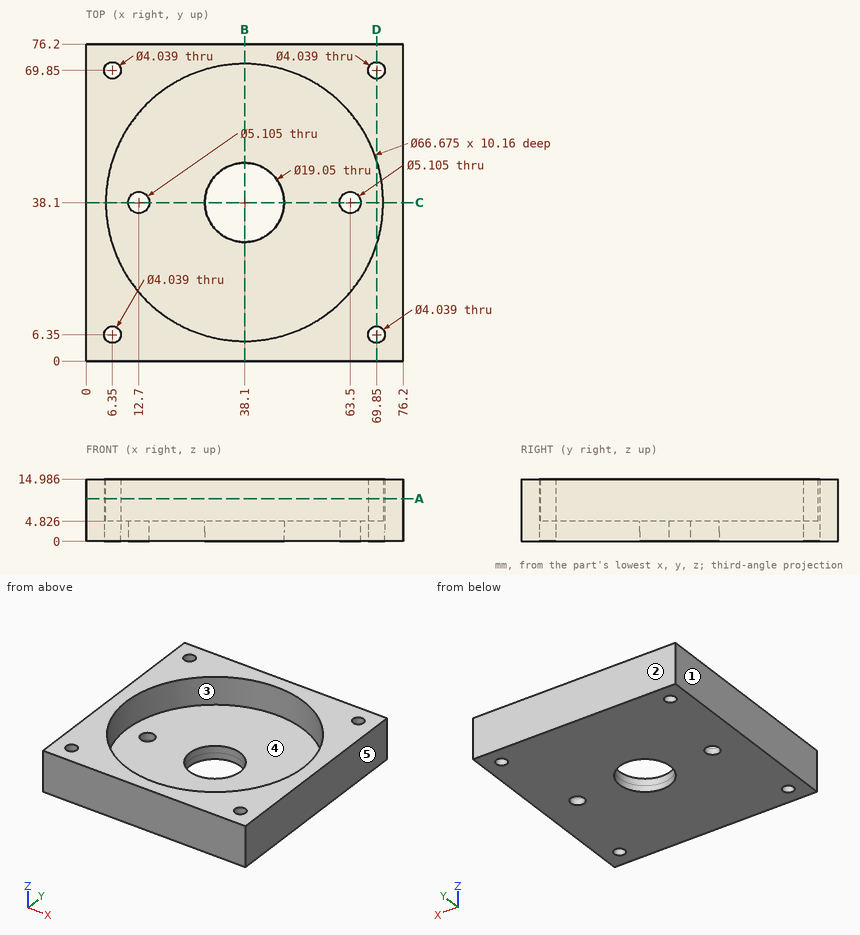
Part print with two shaded views. Sizes in mm from the minimum x, y, z corner. A direction names the side the tool comes from. Give positions to 0.01 mm unless a question says otherwise; leave off trailing zeros. Order: outer loops, then holes, each group sorted by start corner. A loop starts at its lowest first (then second) coordinate and runs counter-clockwise, first axis right, second up.
(1) Drill centre lines: L1, parallel to X at y = 69.85, z = 0.5; L2, parallel to Y at x = 63.5, z = 1.5; L3, parallel to Y at x = 38, z = 7.75. Where is each one in solid material? Low to high.
(2) Mould opens along X. For the marked faces 1, 2 and 3 say: released by +X, released by -X, zero draft, split by the parting line, or undercut.
(3) Flat gauge pins, fed straight in: pin 1 (8 mm diameter, centred on x = 18.5, z = 8, fed in from -Y); pin 2 (8 mm diameter, centred on x = 63.5, y = 38.1, fed in from +Z). Where does each tip first touch, or does it go through?
(4) Saw through at C-C, the plane y = 38.1. Give the cut face in (x, z) (1 decimal).
(5) Saw through at B-B, the plane x = 38.1. Give the cut face in (y, z) (1 decimal).
(6) Saw through at A-A, the plane z = 10.25. State how many separate pieces and enclosed holes the cut face has, then the cut area to 3 significant figures.
(7) Tool access for the marked faces 4 and 5: list every direction of +Z, -Z, +X, -X, +Y, -Y with a clear straight run to the whole face (end or side of a thin tool).
(8) Saw through at D-D, the plane x = 69.85. Give the cut face in (y, z) (1 decimal).
Results found:
1. L1: x = 0 to 4.33, 8.37 to 67.83, 71.87 to 76.2
1. L2: y = 0 to 35.55, 40.65 to 76.2
1. L3: y = 0 to 4.76, 71.44 to 76.2
2. face 1: released by -X
2. face 2: zero draft
2. face 3: undercut
3. pin 1: stops at y = 0
3. pin 2: stops at z = 4.83
4. outline: (0, 0) - (10.1, 0) - (10.1, 4.8) - (4.8, 4.8) - (4.8, 15) - (0, 15) - close; (15.3, 0) - (28.6, 0) - (28.6, 4.8) - (15.3, 4.8) - close; (47.6, 0) - (60.9, 0) - (60.9, 4.8) - (47.6, 4.8) - close; (66.1, 0) - (76.2, 0) - (76.2, 15) - (71.4, 15) - (71.4, 4.8) - (66.1, 4.8) - close
5. outline: (0, 0) - (28.6, 0) - (28.6, 4.8) - (4.8, 4.8) - (4.8, 15) - (0, 15) - close; (47.6, 0) - (76.2, 0) - (76.2, 15) - (71.4, 15) - (71.4, 4.8) - (47.6, 4.8) - close
6. separate pieces: 1
6. enclosed holes: 5
6. area: 2,260 mm2
7. face 4: +Z
7. face 5: +Z, -Z, +X, +Y, -Y
8. outline: (0, 0) - (4.3, 0) - (4.3, 15) - (0, 15) - close; (8.4, 0) - (67.8, 0) - (67.8, 15) - (48.3, 15) - (48.3, 4.8) - (27.9, 4.8) - (27.9, 15) - (8.4, 15) - close; (71.9, 0) - (76.2, 0) - (76.2, 15) - (71.9, 15) - close
